Autodesk Inventor part; units mm, degrees
ref_plane "YZ Plane" through (0, 0, 0) normal (1, 0, 0) x (0, 1, 0)
ref_plane "XZ Plane" through (0, 0, 0) normal (0, 1, 0) x (-1, 0, 0)
ref_plane "XY Plane" through (0, 0, 0) normal (0, 0, 1) x (1, 0, 0)
sketch "Sketch1" plane through (0, 0, 0) normal (0, 0, 1) x (1, 0, 0)
  line L0 (-15, -4) -> (15, -4)
  line L1 (15, -4) -> (15, 4)
  line L2 (15, 4) -> (-15, 4)
  line L3 (-15, 4) -> (-15, -4)
  line L4 (-15, -4) -> (15, 4) construction
  line L5 (15, -4) -> (-15, 4) construction
  point P0 (0, 0)
  dimension "d0" = 8
  dimension "d1" = 30
extrude "Extrusion1" add sketch "Sketch1" along normal blind 15.75 and the other way blind 15.75
sketch "Sketch2" plane through (0, 0, 15.75) normal (0, 0, 1) x (1, 0, 0)
  circle A0 centre (0, 0) radius 1.5
  dimension "d4" = 3
hole "Hole1" at (0, 0, 15.75) direction (0, 0, -1) diameter 3.88 depth 7 countersink diameter 4.34 countersink angle 7
pattern_linear "Rectangular Pattern1" count 2 spacing 10 along (-1, 0, 0) count 2 spacing 10 along (1, 0, 0) of "Hole1"
mirror "Mirror1" about plane through (0, 0, 0) normal (0, 0, 1) of "Hole1", "Rectangular Pattern1"
properties part number "cycloid_base_bottom"
For this review, take the finished solid that the model builds, in its own axes (mm). A direction names the side the tool comes from. Round coordinates to 2 decimals unless told otherwise and drop trailing zeros. Write each loop counter-clockwise with the first axis right and the second up, starting at its lowest first coordinate (ties: lowest second). Pieces come first, ordered by that corner, then holes. Notation, with made-up numbers: (57.25, 56.25) - (105.25, 56.25) arc R13 ccw to (105.25, 72.25) - close; hole circle Ø10 at (63.25, 54). An arc over 180 degrees is marked (long way). Write item = value, one per line. Start each with the question number.
1. Consider section B-B on x = -10. State the section outline as (y, z) points.
2. Consider section A-A on z = 11. State the section outline as (x, y) points.
3. For pin 1 Ø3 at (x, y) = (-10, 0) entering from -Z; pin 2 Ø3 at (x, y) = (10, 0) entering from +Z, all flat-tipped, find the tip position at first contact; note any pin that passes through.
4. For faces 1 (the face through (0, -4, 0)), 2 (the face through (1.9, 0.4, 10.3)), 3 (the face through (0, 0, -8.75)), list the 3-axis set-ups (+Z, -Z, +X, -X, +Y, -Y) from which the entire face can be reached by the end or side of a thin tool; tool diameter is ignored.
5. Wall thickness on L1, parallel to X at y = 0, z = 11.15; L2, parallel to Y at x = 10, z = 11.1; L3, parallel to X at y = -1, z = 12: over which ranges is each line inside the solid? List them lowest first.
6. Draft analysis for pull direction Y (two halves, no side actions). For faces 4 (the face through (0, 4, 0)), 5 (the face through (-10, 0, 8.75)), 6 (the face through (0, 3, -15.75)), state which applies: released by +Y, released by -Y, zero draft, split by the parting line, or undercut.
Evaluation:
q1.outline = (-4, -15.75) - (-2.17, -15.75) - (-1.94, -11.99) - (-1.94, -8.75) - (1.94, -8.75) - (1.94, -11.99) - (2.17, -15.75) - (4, -15.75) - (4, 15.75) - (2.17, 15.75) - (1.94, 11.99) - (1.94, 8.75) - (-1.94, 8.75) - (-1.94, 11.99) - (-2.17, 15.75) - (-4, 15.75) - close
q2.outline = (-15, -4) - (15, -4) - (15, 4) - (-15, 4) - close; hole circle Ø3.88 at (-10, 0); hole circle Ø3.88 at (0, 0); hole circle Ø3.88 at (10, 0)
q3.pin_1 = -8.75
q3.pin_2 = 8.75
q4.face_1 = +Z, -Z, +X, -X, -Y
q4.face_2 = +Z
q4.face_3 = -Z
q5.L1 = -15 to -11.94, -8.06 to -1.94, 1.94 to 8.06, 11.94 to 15
q5.L2 = -4 to -1.94, 1.94 to 4
q5.L3 = -15 to -11.66, -8.34 to -1.66, 1.66 to 8.34, 11.66 to 15
q6.face_4 = released by +Y
q6.face_5 = undercut
q6.face_6 = zero draft
